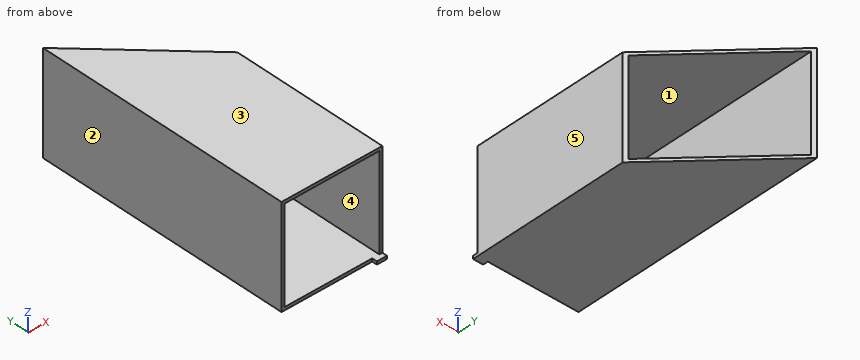
Autodesk Inventor part; units mm, degrees
ref_plane "YZ Plane" through (0, 0, 0) normal (1, 0, 0) x (0, 1, 0)
ref_plane "XZ Plane" through (0, 0, 0) normal (0, 1, 0) x (-1, 0, 0)
ref_plane "XY Plane" through (0, 0, 0) normal (0, 0, 1) x (1, 0, 0)
sketch "Sketch1" plane through (0, 0, 0) normal (0, 1, 0) x (-1, 0, 0)
  line L0 (50, 50) -> (-50, 50)
  line L1 (-50, 50) -> (-50, -50)
  line L2 (-50, -50) -> (50, -50)
  line L3 (50, -50) -> (50, 50)
  line L4 (50, 50) -> (-50, -50) construction
  line L5 (-50, 50) -> (50, -50) construction
  line L6 (47, 47) -> (-47, 47)
  line L7 (-47, 47) -> (-47, -47)
  line L8 (-47, -47) -> (47, -47)
  line L9 (47, -47) -> (47, 47)
  line L10 (47, 47) -> (-47, -47) construction
  line L11 (-47, 47) -> (47, -47) construction
  point P0 (0, 0)
  dimension "d0" = 3
  dimension "d1" = 3
  dimension "d2" = 100
  dimension "d3" = 100
extrude "Extrusion1" add sketch "Sketch1" along normal blind 255
sketch "Sketch2" plane through (-50, 0, 50) normal (0, 0, 1) x (1, 0, 0)
  line L0 (0, 0) -> (100, 0)
  line L1 (100, 0) -> (100, 255)
  line L2 (0, 255) -> (100, 255)
  line L3 (0, 0) -> (0, 255)
  line L4 (0, 255) -> (100, 155)
  point P0 (50, 0)
  dimension "d6" = 45
extrude "Extrusion2" cut sketch "Sketch2" against normal through all contours L2 L1 L4
sketch "Sketch3" plane through (0, 0, 0) normal (0, -1, 0) x (1, 0, 0)
  line L0 (-47, -47) -> (-47, 47)
  line L1 (-50, -50) -> (-50, 50)
  line L2 (-47, 25) -> (-50, 25)
  line L3 (-50, 25) -> (-50, 22)
  line L4 (-50, 22) -> (-47, 22)
  line L5 (-47, 22) -> (-47, 25)
  line L6 (50, -50) -> (50, 50)
  line L7 (50, -47) -> (40, -47)
  line L8 (40, -47) -> (40, -50)
  line L9 (40, -50) -> (50, -50)
  line L10 (50, -50) -> (50, -47)
  line L11 (50, 50) -> (50, -50)
  line L12 (-50, 50) -> (50, 50)
  line L13 (-50, -50) -> (-50, 50)
  line L14 (50, -50) -> (-50, -50)
  line L15 (-47, 47) -> (-47, -47)
  line L16 (47, 47) -> (-47, 47)
  line L17 (47, -47) -> (47, 47)
  line L18 (-47, -47) -> (47, -47)
  line L19 (50, -50) -> (-50, -50)
  point P0 (0, 0)
  point P1 (-48.5, 25)
  dimension "d9" = 10
  dimension "d10" = 3
  dimension "d11" = 25
extrude "Extrusion3" add sketch "Sketch3" along normal blind 5 contours L7 L6 L9 L8
properties part number "WI-ShaftRS3" material "Steel"
Read the model definition and answer for the solid it produces. Units are mm, in the model's axes. Face numbers are marked on the shaded views. A direction names the side the tool comes from. Give positions to 0.01 mm unless a question says otherwise; leave off trailing zeros. Order: outer loops, then holes, each group sorted by start corner. A loop starts at its lowest first (then second) coordinate and runs counter-clockwise, first axis right, second up. Notation, with made-up numbers: (82.5, -3.5) -> (108.5, -3.5) arc R5 cw to (108.5, 1.5) -> close; hole circle Ø3 at (-29.5, 23.5). An arc over 180 degrees is marked (long way). One line per item, written item: value. Start each with the question number.
(1) The part is cut by section C-C (z = 36.5). Determine the outline of the cut face in (x, y), and give its area (3 significant figures).
(2) Flat-ended cylindrical pins translate along their axes: P1, Ø1.5, axis at y = 208, z = 23.5, coming from the +X side; P2, Ø2.5, axis at y = -3, z = -49, coming from the -X side. Find the tip coordinate at first contact, or state that the pin passes through.
(3) For a pull along Z with two mould halves and no side action, classify the marked faces 1, 2 and 3 as released by +Z, released by -Z, zero draft, split by the parting line, or undercut.
(4) The part is cut by section D-D (y = 184.5). Determine the outline of the cut face in (x, z), and give its area (3 significant figures).
(5) Straight lines are drawn through the part: L1, parallel to Z at x = -28.5, y = 64; L2, parallel to X at y = 194, z = 1. For each, find the intervals that lie inside material, in ascending order.
(6) The part is cut by section B-B (y = 128.5). Determine the outline of the cut face in (x, z).
(7) The part is cut by section A-A (x = 23.5). Determine the outline of the cut face in (y, z).
(8) A tool of negligible diameter and unlimited length cuts with its end or side. For the marked faces 4 and 5, from which of +Z, -Z, +X, -X, +Y, -Y can it reach the whole face along a straight path? Write none if from no direction.
Taken from the geometry:
1. outline: (-50, 0) -> (-47, 0) -> (-47, 252) -> (-50, 255) -> close; (47, 0) -> (50, 0) -> (50, 155) -> (47, 158) -> close
1. area: 1,230 mm^2
2. P1: x = -47
2. P2: x = 40
3. face 1: undercut
3. face 2: zero draft
3. face 3: released by +Z
4. outline: (-50, -50) -> (20.5, -50) -> (20.5, -47) -> (-47, -47) -> (-47, 47) -> (20.5, 47) -> (20.5, 50) -> (-50, 50) -> close
4. area: 705 mm^2
5. L1: -50 to -47, 47 to 50
5. L2: -50 to -47
6. outline: (-50, -50) -> (50, -50) -> (50, 50) -> (-50, 50) -> close; hole (-47, -47) -> (47, -47) -> (47, 47) -> (-47, 47) -> close
7. outline: (0, -50) -> (181.5, -50) -> (181.5, -47) -> (0, -47) -> close; (0, 47) -> (181.5, 47) -> (181.5, 50) -> (0, 50) -> close
8. face 4: +Y, -Y
8. face 5: +Z, -Z, +X, +Y, -Y
